```python
from build123d import *

# Parameters (mm, degrees)
F1_DEPTH = 9
F2_R     = 22.5
F3_DEPTH = 9.001
F4_R     = 53.1126983722
F5_SIZE  = 10


with BuildPart() as f1:
    # F0 (on Front) → F1 (new body)
    with BuildSketch(Plane.XZ):
        Polygon((-290, 0), (0, 0), (0, 190), (-180, 190), (-180, 120), (-290, 120), align=None)
    extrude(amount=F1_DEPTH)

    # F2 (on Front) → F3 (cut, through all)
    with BuildSketch(Plane.XZ):
        with BuildLine():
            Line((-32, 176), (-82, 176))
            ThreePointArc((-82, 176), (-88, 170), (-82, 164))
            Line((-82, 164), (-32, 164))
            ThreePointArc((-32, 164), (-26, 170), (-32, 176))
        make_face()
        with BuildLine():
            Line((-32, 136), (-82, 136))
            ThreePointArc((-82, 136), (-88, 130), (-82, 124))
            Line((-82, 124), (-32, 124))
            ThreePointArc((-32, 124), (-26, 130), (-32, 136))
        make_face()
        with Locations((-250, 60)):
            Circle(F2_R)
    extrude(amount=F3_DEPTH, mode=Mode.SUBTRACT)

    # F4
    f4_edges = [f1.edges().sort_by_distance(p)[0] for p in [
        (-180, -4.5, 120),
    ]]
    fillet(f4_edges, radius=F4_R)

    # F5
    f5_edges = [f1.edges().sort_by_distance(p)[0] for p in [
        (-290, -4.5, 0),
        (-290, -4.5, 120),
    ]]
    chamfer(f5_edges, length=F5_SIZE)


solid = f1.part
```
The model under review builds one solid part; all positions refer to its coordinate system, in mm. A direction names the side the tool comes from. Give positions to 0.01 mm unless a question says otherwise; leave off trailing zeros. Write each loop counter-clockwise with the first axis right and the second up, starting at its lowest first coordinate (ties: lowest second). Pieces come first, ordered by that corner, then holes. Notation, with made-up numbers: M 80,-1 L 96,-1 A19 cw 96,3 Z; hole C 56.5,58 d3. An arc over 180 degrees is marked long. Write item = value, one per line. Start each with the question number.
Q1. Clearance check with a flat-ended pin moving along its axis: pin 1 (4.5 mm diameter, centred on x = -256, y = -4.5, fed in from +Z). State where the tip first meets the part, or that it passes through.
Q2. For line 1 (Z direction, x = -32, y = -7); line 2 (Z direction, x = -250, y = -3.5); line 3 (X direction, y = -4.25, z = 60), list the stretches that pass through material, from the lowest coordinate up.
Q3. Mouldability with a two-part tool opening along Z and no side actions: class faces 4 (the face through (-88, -4, 130)), 5 (the face through (-57, -4, 136)), 6 (the face through (-147, 0, 96)), 7 (the face through (-89, -4, 190)) as released by +Z, released by -Z, zero draft, split by the parting line, or undercut.
Q4. We need section B-B (z = 60). State the section outline as (x, y) points, plus the area to 4 significant figures.
Q5. We need section A-A (x = -250). State the section outline as (y, z) points, plus the area to 3 significant figures.
Q6. We need section D-D (y = -2.5). State the section outline as (x, z) points.
Q7. Machinability: for faces 1 (the face through (-180, -4, 182)), 2 (the face through (-290, -4, 61)), 3 (the face through (-26, -4, 130)), which of the approach directions +Z, -Z, +X, -X, +Y, -Y give a long, thin tool a straight path to every point of the face, cutting with its end or side? Answer none if there is none.
Q8. We need section C-C (x = -36.5). State the section outline as (y, z) points, plus the area to 3 significant figures.
Result set:
q1.pin_1 = 120
q2.line_1 = 0 to 124, 136 to 164, 176 to 190
q2.line_2 = 0 to 37.5, 82.5 to 120
q2.line_3 = -290 to -272.5, -227.5 to 0
q3.face_4 = undercut
q3.face_5 = undercut
q3.face_6 = zero draft
q3.face_7 = released by +Z
q4.outline = M -290,-9 L -272.5,-9 L -272.5,0 L -290,0 Z; M -227.5,-9 L 0,-9 L 0,0 L -227.5,0 Z
q4.area = 2,205 mm2
q5.outline = M -9,0 L 0,0 L 0,37.5 L -9,37.5 Z; M -9,82.5 L 0,82.5 L 0,120 L -9,120 Z
q5.area = 675 mm2
q6.outline = M -290,10 L -280,0 L 0,0 L 0,190 L -180,190 L -180,173.11 A53.11 cw -233.11,120 L -280,120 L -290,110 Z; hole C -250,60 d45; hole M -82,124 L -32,124 A6 ccw -32,136 L -82,136 A6 ccw Z; hole M -82,164 L -32,164 A6 ccw -32,176 L -82,176 A6 ccw Z
q7.face_1 = +Z, -X, +Y, -Y
q7.face_2 = +Z, -Z, -X, +Y, -Y
q7.face_3 = +Y, -Y
q8.outline = M -9,0 L 0,0 L 0,124 L -9,124 Z; M -9,136 L 0,136 L 0,164 L -9,164 Z; M -9,176 L 0,176 L 0,190 L -9,190 Z
q8.area = 1,490 mm2
